from build123d import *

# Parameters (mm, degrees)
CROQUIS1_W              = 60
CROQUIS1_H              = 65
CROQUIS1_R              = 3
SALIENTE_EXTRUIR1_DEPTH = 2.9
REDONDEO2_R             = 5
REDONDEO3_R             = 5
REDONDEO4_R             = 5
REDONDEO5_R             = 5


with BuildPart() as part:
    # Croquis1 → Saliente-Extruir1 (new body)
    with BuildSketch(Plane.XY):
        with Locations((30, 32.5)):
            Rectangle(CROQUIS1_W, CROQUIS1_H)
        with Locations((42, 42.5)):
            Circle(CROQUIS1_R, mode=Mode.SUBTRACT)
    extrude(amount=-SALIENTE_EXTRUIR1_DEPTH)

    # Redondeo2
    redondeo2_edges = [part.edges().sort_by_distance(p)[0] for p in [
        (0, 65, -1.45),
    ]]
    fillet(redondeo2_edges, radius=REDONDEO2_R)

    # Redondeo3
    redondeo3_edges = [part.edges().sort_by_distance(p)[0] for p in [
        (60, 65, -1.45),
    ]]
    fillet(redondeo3_edges, radius=REDONDEO3_R)

    # Redondeo4
    redondeo4_edges = [part.edges().sort_by_distance(p)[0] for p in [
        (60, 0, -1.45),
    ]]
    fillet(redondeo4_edges, radius=REDONDEO4_R)

    # Redondeo5
    redondeo5_edges = [part.edges().sort_by_distance(p)[0] for p in [
        (0, 0, -1.45),
    ]]
    fillet(redondeo5_edges, radius=REDONDEO5_R)


solid = part.part
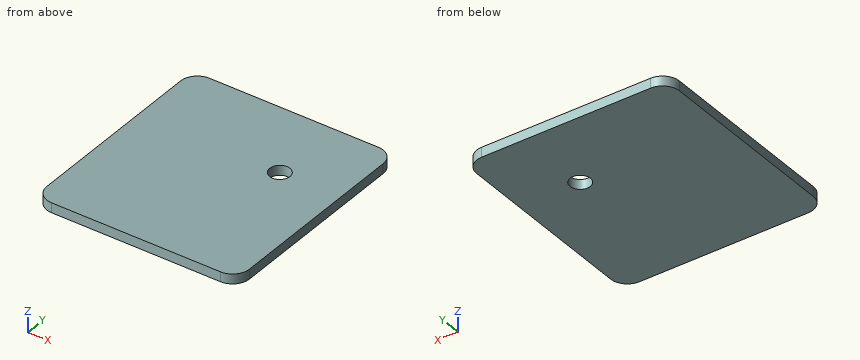
Geometry check sheet. Reference: the model listing, model coordinates, mm. Give positions to 0.01 mm unless a question says otherwise; leave off trailing zeros. Loops run counter-clockwise (first coordinate to the right, second up) from the corner with the lowest first, then second, coordinate; pieces in that order, holes last. Notation, with made-up numbers: M 70.25,83.5 L 78.25,83.5 A18 ccw 78.25,106.5 Z; hole C 26,-28.5 d9. An arc over 180 degrees is marked long. Answer as a JSON object with one key per item and string values. Group by question number.
Item 1: Sectioned sample at B-B on x = 42. Record the boundary of the cut face in (y, z).
Item 2: Material ranges on L1, parallel to Y at x = 42, z = -1.85; L2, parallel to Y at x = 40, z = -2.05; L3, parallel to X at y = 44, z = -1.8, recorded low to high.
Item 3: Sectioned sample at A-A on y = 42.5. Record the boundary of the cut face in (x, z).
Findings below:
{
 "1": {"outline": "M 0,-2.9 L 39.5,-2.9 L 39.5,0 L 0,0 Z; M 45.5,-2.9 L 65,-2.9 L 65,0 L 45.5,0 Z"},
 "2": {"L1": "0 to 39.5, 45.5 to 65", "L2": "0 to 40.26, 44.74 to 65", "L3": "0 to 39.4, 44.6 to 60"},
 "3": {"outline": "M 0,-2.9 L 39,-2.9 L 39,0 L 0,0 Z; M 45,-2.9 L 60,-2.9 L 60,0 L 45,0 Z"}
}
